Autodesk Inventor part; units mm, degrees
ref_plane "YZ Plane" through (0, 0, 0) normal (1, 0, 0) x (0, 1, 0)
ref_plane "XZ Plane" through (0, 0, 0) normal (0, 1, 0) x (-1, 0, 0)
ref_plane "XY Plane" through (0, 0, 0) normal (0, 0, 1) x (1, 0, 0)
sketch "Sketch1" plane through (0, 0, 0) normal (0, 0, 1) x (1, 0, 0)
  line L0 (0, 5.6) -> (0, -4.2)
  line L1 (-9.6, 0) -> (12.8, 0)
  line L2 (-8, 3.5) -> (8, 3.5)
  line L3 (8, 3.5) -> (8, -3.5)
  line L4 (8, -3.5) -> (-8, -3.5)
  line L5 (-8, -3.5) -> (-8, 3.5)
  dimension "d0" = 16
  dimension "d1" = 7
extrude "Extrusion1" add sketch "Sketch1" along normal blind 8
sketch "Sketch2" plane through (0, 0, 8) normal (0, 0, 1) x (1, 0, 0)
  line L0 (8, 3.5) -> (8, -3.5)
  line L1 (-6, 2.5) -> (7, 2.5)
  line L2 (7, 2.5) -> (7, -2)
  line L3 (7, -2) -> (-6, -2)
  line L4 (-6, -2) -> (-6, 2.5)
  line L5 (-4, -2) -> (4, -2)
  line L6 (4, -2) -> (4, -2.5)
  line L7 (4, -2.5) -> (-4, -2.5)
  line L8 (-4, -2.5) -> (-4, -2)
  line L9 (-6, 1.25) -> (-7, 1.25)
  line L10 (-7, 1.25) -> (-7, -1.25)
  line L11 (-7, -1.25) -> (-6, -1.25)
  line L12 (-6, -1.25) -> (-6, 1.25)
  line L13 (0, 5.6) -> (0, -4.2)
  line L14 (-9.6, 0) -> (12.8, 0)
  dimension "d4" = 14
  dimension "d5" = 1
  dimension "d6" = 2.5
  dimension "d7" = 0.5
  dimension "d8" = 5
  dimension "d9" = 1
  dimension "d10" = 8
extrude "Extrusion2" cut sketch "Sketch2" against normal blind 6
sketch "Sketch3" plane through (0, 0, 2) normal (0, 0, 1) x (1, 0, 0)
  line L0 (0, 5.6) -> (0, -4.2)
  line L1 (-9.6, 0) -> (12.8, 0)
  line L2 (-3.25, 0) -> (3.25, 0)
  line L3 (3.25, 0) -> (3.25, -0.25)
  line L4 (3.25, -0.25) -> (-3.25, -0.25)
  line L5 (-3.25, -0.25) -> (-3.25, 0)
  line L6 (3.25, 0) -> (3, 0)
  line L7 (3, 0) -> (3, 1.75)
  line L8 (3, 1.75) -> (3.25, 1.75)
  line L9 (3.25, 1.75) -> (3.25, 0)
  dimension "d13" = 6.5
  dimension "d14" = 2
  dimension "d15" = 0.25
  dimension "d16" = 0.25
extrude "Extrusion3" add sketch "Sketch3" along normal blind 5.5
sketch "Sketch4" plane through (0, 0, 2) normal (0, 0, 1) x (1, 0, 0)
  line L0 (-3.25, 0) -> (3, 0)
  line L1 (3, 0) -> (3, 1.75)
  line L2 (2.7, 0) -> (2.3, 0)
  line L3 (2.3, 0) -> (2.3, 0.5)
  line L4 (2.3, 0.5) -> (2.7, 0.5)
  line L5 (2.7, 0.5) -> (2.7, 0)
  dimension "d19" = 0.3
  dimension "d20" = 0.4
  dimension "d21" = 0.5
extrude "Extrusion4" cut sketch "Sketch4" against normal blind 0.5
pattern_linear "Rectangular Pattern1" count 6 spacing 1 along (-1, 0, 0) of "Extrusion4"
equation "\"d15\" = d16"
properties part number "config - j9h2 connector"
For this review, take the finished solid that the model builds, in its own axes (mm). A direction names the side the tool comes from. Coordinates: 2 decimals unless noted, no trailing zeros. Write each loop counter-clockwise with the first axis right and the second up, starting at its lowest first coordinate (ties: lowest second). Pieces come first, ordered by that corner, then holes.
(1) Wall thickness on probe 1 along Y at (x, z) = (2, 6.75); probe 2 along X at (y, z) = (0.75, 7.25); probe 3 along Y at (x, z) = (-4.25, 7): over which ranges is each line inside the solid? List them lowest first.
(2) Tool access review of faces 5 (the face through (-8, 0, 4)), 6 (the face through (0, 2.5, 5)): name each direction out of +Z, -Z, +X, -X, +Y, -Y from which nothing blocks a thin tool from reaching the whole face with its end or side.
(3) Add section A-A on z = 7.25. Give the boundary of the cut face in (x, y).
(4) For pin 1 Ø1.5 at (x, y) = (4.5, 1.5) entering from +Z, flat-tipped, find the tip position at first contact; note if it passes through.
(5) Add section B-B on y = 2. Give the boundary of the cut face in (x, z).
(6) The part is to be moulded in two halves that separate along Y. For faces 1 (the face through (0, -3.5, 4)), 2 (the face through (0, 3.5, 4)), 3 (the face through (6, -2, 5)), 4 (the face through (8, 0, 4)), say which applies: +Y half, -Y half, draft (parallel to the pull), parting line (faces both ways), or undercut.
(7) Add section C-C on x = -6.75. Give the boundary of the cut face in (y, z).
Answer sheet:
1. probe 1: y = -3.5 to -2.5, -0.25 to 0, 2.5 to 3.5
1. probe 2: x = -8 to -7, 3 to 3.25, 7 to 8
1. probe 3: y = -3.5 to -2, 2.5 to 3.5
2. face 5: +Z, -Z, -X, +Y, -Y
2. face 6: +Z
3. outline: (-8, -3.5) - (8, -3.5) - (8, 3.5) - (-8, 3.5) - close; (-3.25, -0.25) - (3.25, -0.25) - (3.25, 1.75) - (3, 1.75) - (3, 0) - (-3.25, 0) - close; hole (-7, -1.25) - (-6, -1.25) - (-6, -2) - (-4, -2) - (-4, -2.5) - (4, -2.5) - (4, -2) - (7, -2) - (7, 2.5) - (-6, 2.5) - (-6, 1.25) - (-7, 1.25) - close
4. pin 1: stops at z = 2
5. outline: (-8, 0) - (8, 0) - (8, 8) - (7, 8) - (7, 2) - (-6, 2) - (-6, 8) - (-8, 8) - close
6. face 1: -Y half
6. face 2: +Y half
6. face 3: undercut
6. face 4: draft
7. outline: (-3.5, 0) - (3.5, 0) - (3.5, 8) - (1.25, 8) - (1.25, 2) - (-1.25, 2) - (-1.25, 8) - (-3.5, 8) - close
